The listing builds one solid part. Answer for the finished solid, in the listing's coordinates (mm). A direction names the side the tool comes from. Round coordinates to 2 decimals unless told otherwise and drop trailing zeros. Order: outer loops, then holes, each group sorted by start corner. A loop starts at its lowest first (then second) coordinate and runs counter-clockwise, first axis right, second up. Notation, with made-up numbers: (-39, 40.5) -> (-30, 40.5) arc R29 cw to (-30, 69.5) -> close; hole circle Ø8 at (-37, -19.5). An arc over 180 degrees is marked (long way). Return JSON: item names as keys, results as strings. Group by question number.
(1) Consider line 1 (X direction, y = 0, z = 2.2) (3 decimals); line 2 (X direction, y = -0.25, z = 0.5). Determine where each line is inside the solid, lowest interval first. Write a range as [from, to].
(2) Each of these flat-tipped pins is pushed along its axis until it touches: pin 1 (4 mm diameter, centred on x = -1, y = 0, fed in from -Z); pin 2 (1 mm diameter, centred on x = 4, y = -4, fed in from -Z); pin 3 (1.6 mm diameter, centred on x = -4, y = 3.5, fed in from -Z). Where does it stop, or does it pass through?
(3) The part is cut by section C-C (y = 0). Determine the outline of the cut face in (x, z) (3 decimals).
(4) The part is cut by section A-A (z = 7.5). Determine the outline of the cut face in (x, y) (3 decimals).
(5) Determine the mould class of faces 1 (the face through (7, 0, 0)), 2 (the face through (0, 7.9, 5)), 3 (the face through (4, -4, 10)) for opening direction Y: +Y half, -Y half, draft (parallel to the pull), parting line (faces both ways), or undercut.
(6) Which of the six approach directions +Z, -Z, +X, -X, +Y, -Y give full straight-line access (tool end or side, diameter ignored) to faces 4 (the face through (0, -6.5, 4)), 5 (the face through (3.65, 6.38, 10.48)), 6 (the face through (-4, 4, 11.4))?
(7) The part is cut by section B-B (z = 1.25). Determine the outline of the cut face in (x, y) (3 decimals).
from build123d import *

# Parameters (mm, degrees)
F1_W     = 15.8
F1_H     = 15.8
F2_DEPTH = 9.58
F0_R     = 2.4150125628
F0_R_2   = 2.435
F3_DEPTH = 11.4
F4_T     = -1.4
F5_R     = 3.135
F6_DEPTH = 7.54
F7_R     = 2.415
F8_DEPTH = 4.7


with BuildPart() as f2:
    # F1 (on Top) → F2 (new body)
    with BuildSketch(Plane.XY):
        Rectangle(F1_W, F1_H)
    extrude(amount=F2_DEPTH)

    # F0 (on Top) → F3 (join)
    with BuildSketch(Plane.XY):
        with Locations((-3.9849874372, 3.9849874372)):
            Circle(F0_R)
        with Locations((3.965, 3.965)):
            Circle(F0_R_2)
        with Locations((3.965, -3.965)):
            Circle(F0_R_2)
        with Locations((-3.9849874372, -3.9849874372)):
            Circle(F0_R)
    extrude(amount=F3_DEPTH)

    # F4
    f4_openings = [f2.faces().sort_by_distance(p)[0] for p in [
        (0, 0, 0),
    ]]
    offset(amount=F4_T, openings=f4_openings, kind=Kind.INTERSECTION)

    # F5 (on face) → F6 (join)
    with BuildSketch(Plane(origin=(0, 0, 8.18), x_dir=(1, 0, 0), z_dir=(0, 0, -1))):
        Circle(F5_R)
    extrude(amount=F6_DEPTH)

    # F7 (on face) → F8 (cut)
    with BuildSketch(Plane(origin=(0, 0, 0.64), x_dir=(1, 0, 0), z_dir=(0, 0, -1))):
        Circle(F7_R)
    extrude(amount=-F8_DEPTH, mode=Mode.SUBTRACT)


solid = f2.part
Answer below:
{
 "1": {"line 1": "x = [-7.9, -6.5], [-3.135, -2.415], [2.415, 3.135], [6.5, 7.9]", "line 2": "x = [-7.9, -6.5], [6.5, 7.9]"},
 "2": {"pin 1": "stops at z = 0.64", "pin 2": "stops at z = 10", "pin 3": "stops at z = 8.18"},
 "3": {"outline": "(-7.9, 0) -> (-6.5, 0) -> (-6.5, 8.18) -> (-3.135, 8.18) -> (-3.135, 0.64) -> (-2.415, 0.64) -> (-2.415, 5.34) -> (2.415, 5.34) -> (2.415, 0.64) -> (3.135, 0.64) -> (3.135, 8.18) -> (6.5, 8.18) -> (6.5, 0) -> (7.9, 0) -> (7.9, 9.58) -> (-7.9, 9.58) -> close"},
 "4": {"outline": "(-7.9, -7.9) -> (7.9, -7.9) -> (7.9, 7.9) -> (-7.9, 7.9) -> close; circle Ø6.27 at (0, 0); hole (-6.5, -6.5) -> (6.5, -6.5) -> (6.5, 6.5) -> (-6.5, 6.5) -> close"},
 "5": {"face 1": "draft", "face 2": "+Y half", "face 3": "undercut"},
 "6": {"face 4": "-Z", "face 5": "+Z", "face 6": "+Z, +X, -X, +Y, -Y"},
 "7": {"outline": "(-7.9, -7.9) -> (7.9, -7.9) -> (7.9, 7.9) -> (-7.9, 7.9) -> close; circle Ø6.27 at (0, 0); hole (-6.5, -6.5) -> (6.5, -6.5) -> (6.5, 6.5) -> (-6.5, 6.5) -> close; hole circle Ø4.83 at (0, 0)"}
}
